Build history of the part. All positions in model axes, mm. Face numbers are marked on the shaded views. Round coordinates to 2 decimals unless told otherwise and drop trailing zeros. Order: outer loops, then holes, each group sorted by start corner. A loop starts at its lowest first (then second) coordinate and runs counter-clockwise, first axis right, second up. Notation, with made-up numbers: (1.25, 4.5) -> (46.25, 4.5) arc R16 ccw to (46.25, 12.5) -> close; hole circle Ø4 at (89.5, 53.25). An arc over 180 degrees is marked (long way). Use a Markdown table: item, result. Add a question column.
Item 1: Probe L1, parallel to Z at x = -71.5, y = 17; L2, parallel to Y at x = -71, z = 40.5; L3, parallel to X at y = 31, z = -36. List the from-to ranges inside material, lowest first.
Item 2: Two-plate mould, pull along Y, no slides. Class the marked faces 1, 2 and 3: released by +Y, released by -Y, zero draft, split by the parting line, or undercut.
Item 3: Slice it at B-B, the plane z = -17. Give the cut face in (x, y).
Item 4: Slice it at D-D, the plane z = -52. Give the cut face in (x, y), plus the area to 3 significant figures.
Item 5: Pin check, flat tips, straight feed: pin 1 (2 mm diameter, centred on x = -27.5, z = -48, fed in from -Y); pin 2 (4 mm diameter, centred on y = 40, z = -45.5, fed in from +X); pin 3 (4 mm diameter, centred on y = 40.5, z = -26.5, fed in from -X); pin 4 (23 mm diameter, centred on y = 45, z = -16, fed in from +X). Stop position of each tip, or through.
Item 6: Slice it at C-C, the plane y = 41. Give the cut face in (x, z).
Item 7: Slice it at A-A, the plane y = 4.5. Give the cut face in (x, z).
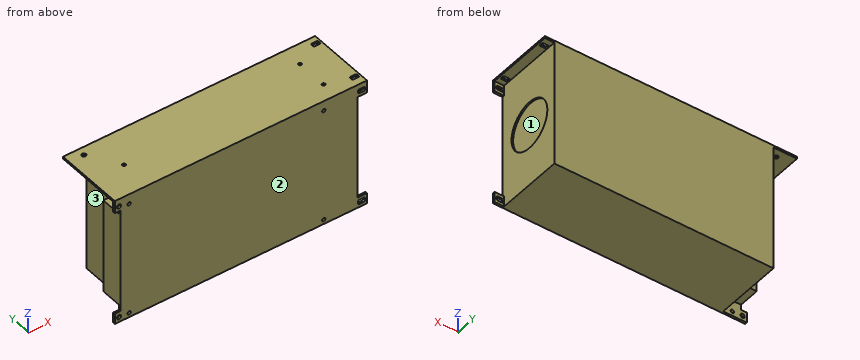
from build123d import *

# Parameters (mm, degrees)
SZKIC1_W                    = 240
SZKIC1_H                    = 122
DODANIE_WYCI_GNI_CIE1_DEPTH = 2
SZKIC2_W                    = 240
SZKIC2_H                    = 2
DODANIE_WYCI_GNI_CIE2_DEPTH = 64
SZKIC3_W                    = 9.1
SZKIC3_H                    = 99.9
SZKIC3_W_2                  = 5.5
WYTNIJ_WYCI_GNI_CIE1_DEPTH  = 180.195703173
SZKIC4_W                    = 208.5
SZKIC4_H                    = 120
DODANIE_WYCI_GNI_CIE3_DEPTH = 64
SZKIC5_R                    = 22.806294832
WYTNIJ_WYCI_GNI_CIE2_DEPTH  = 1.5
SZKIC6_W                    = 16.9
SZKIC6_H                    = 90.349503158
DODANIE_WYCI_GNI_CIE4_DEPTH = 20
WYTNIJ_WYCI_GNI_CIE3_DEPTH  = 180.195703173
SZKIC8_R                    = 2
WYTNIJ_WYCI_GNI_CIE4_DEPTH  = 180.195703173
SZKIC9_R                    = 1.6
SZKIC9_R_2                  = 1.651116854
WYTNIJ_WYCI_GNI_CIE5_DEPTH  = 2
SZKIC10_R                   = 2
WYTNIJ_WYCI_GNI_CIE6_DEPTH  = 2
SZKIC11_R                   = 1.455539738
SZKIC11_R_2                 = 1.5
WYTNIJ_WYCI_GNI_CIE7_DEPTH  = 2


with BuildPart() as part:
    # Szkic1 → Dodanie-wyciągnięcie1 (new body)
    with BuildSketch(Plane(origin=(0, 0, 0), x_dir=(1, 0, 0), z_dir=(0, 1, 0))):
        with Locations((29.433962264, 14.396226415)):
            Rectangle(SZKIC1_W, SZKIC1_H)
    extrude(amount=DODANIE_WYCI_GNI_CIE1_DEPTH)

    # Szkic2 → Dodanie-wyciągnięcie2 (add)
    with BuildSketch(Plane(origin=(0, 2, 0), x_dir=(1, 0, 0), z_dir=(0, 1, 0))):
        with Locations((29.433962264, -45.603773585)):
            Rectangle(SZKIC2_W, SZKIC2_H)
    extrude(amount=DODANIE_WYCI_GNI_CIE2_DEPTH)

    # Szkic3 → Wytnij-wyciągnięcie1 (cut, through all)
    with BuildSketch(Plane(origin=(0, 2, 0), x_dir=(1, 0, 0), z_dir=(0, 1, 0))):
        with Locations((144.883962264, 15.346226415)):
            Rectangle(SZKIC3_W, SZKIC3_H)
        with Locations((-87.816037736, 15.346226415)):
            Rectangle(SZKIC3_W_2, SZKIC3_H)
    extrude(amount=-WYTNIJ_WYCI_GNI_CIE1_DEPTH, mode=Mode.SUBTRACT)

    # Szkic4 → Dodanie-wyciągnięcie3 (add)
    with BuildSketch(Plane(origin=(0, 2, 0), x_dir=(1, 0, 0), z_dir=(0, 1, 0))):
        with Locations((36.083962264, 15.396226415)):
            Rectangle(SZKIC4_W, SZKIC4_H)
    extrude(amount=DODANIE_WYCI_GNI_CIE3_DEPTH)

    # Szkic5 → Wytnij-wyciągnięcie2 (cut)
    with BuildSketch(Plane(origin=(140.333962264, 0, 0), x_dir=(0, 0, -1), z_dir=(1, 0, 0))):
        with Locations((16.047891544, 34.239354483)):
            Circle(SZKIC5_R)
    extrude(amount=-WYTNIJ_WYCI_GNI_CIE2_DEPTH, mode=Mode.SUBTRACT)

    # Szkic6 → Dodanie-wyciągnięcie4 (add)
    with BuildSketch(Plane(origin=(0, 2, 0), x_dir=(1, 0, 0), z_dir=(0, 1, 0))):
        with Locations((-76.616037736, 15.234150699)):
            Rectangle(SZKIC6_W, SZKIC6_H)
    extrude(amount=DODANIE_WYCI_GNI_CIE4_DEPTH)

    # Szkic7 → Wytnij-wyciągnięcie3 (cut, through all)
    with BuildSketch(Plane(origin=(0, 2, 0), x_dir=(1, 0, 0), z_dir=(0, 1, 0))):
        with BuildLine():
            Line((141.913386631, 72.496226415), (146.454537897, 72.496226415))
            ThreePointArc((146.454537897, 72.496226415), (147.147095509, 72.20935966), (147.433962264, 71.516802048))
            Line((147.433962264, 71.516802048), (147.433962264, 69.275650782))
            ThreePointArc((147.433962264, 69.275650782), (147.147095509, 68.583093171), (146.454537897, 68.296226415))
            Line((146.454537897, 68.296226415), (141.913386631, 68.296226415))
            ThreePointArc((141.913386631, 68.296226415), (141.22082902, 68.583093171), (140.933962264, 69.275650782))
            Line((140.933962264, 69.275650782), (140.933962264, 71.516802048))
            ThreePointArc((140.933962264, 71.516802048), (141.22082902, 72.20935966), (141.913386631, 72.496226415))
        make_face()
        with BuildLine():
            Line((141.913386631, -37.603773585), (146.454537897, -37.603773585))
            ThreePointArc((146.454537897, -37.603773585), (147.147095509, -37.89064034), (147.433962264, -38.583197952))
            Line((147.433962264, -38.583197952), (147.433962264, -40.424349218))
            ThreePointArc((147.433962264, -40.424349218), (147.147095509, -41.116906829), (146.454537897, -41.403773585))
            Line((146.454537897, -41.403773585), (141.913386631, -41.403773585))
            ThreePointArc((141.913386631, -41.403773585), (141.22082902, -41.116906829), (140.933962264, -40.424349218))
            Line((140.933962264, -40.424349218), (140.933962264, -38.583197952))
            ThreePointArc((140.933962264, -38.583197952), (141.22082902, -37.89064034), (141.913386631, -37.603773585))
        make_face()
    extrude(amount=-WYTNIJ_WYCI_GNI_CIE3_DEPTH, mode=Mode.SUBTRACT)

    # Szkic8 → Wytnij-wyciągnięcie4 (cut, through all)
    with BuildSketch(Plane(origin=(0, 2, 0), x_dir=(1, 0, 0), z_dir=(0, 1, 0))):
        with Locations(Location((-86.566037736, 70.596226415, 0), (0, 0, 270))):
            Circle(SZKIC8_R)
        with Locations(Location((-86.566037736, -39.353773585, 0), (0, 0, 270))):
            Circle(SZKIC8_R)
    extrude(amount=-WYTNIJ_WYCI_GNI_CIE4_DEPTH, mode=Mode.SUBTRACT)

    # Szkic9 → Wytnij-wyciągnięcie5 (cut)
    with BuildSketch(Plane.XZ):
        with Locations(Location((-76.966037736, 37.203773585, 0), (0, 0, 270))):
            Circle(SZKIC9_R)
        with Locations(Location((108.333962264, 37.203773585, 0), (0, 0, 270))):
            Circle(SZKIC9_R)
        with Locations(Location((108.333962264, -70.996226415, 0), (0, 0, 270))):
            Circle(SZKIC9_R)
        with Locations(Location((-76.914920882, -71.047343269, 0), (0, 0, 270))):
            Circle(SZKIC9_R_2)
    extrude(amount=-WYTNIJ_WYCI_GNI_CIE5_DEPTH, mode=Mode.SUBTRACT)

    # Szkic10 → Wytnij-wyciągnięcie6 (cut)
    with BuildSketch(Plane.XY.offset(46.603773585)):
        with Locations((-76.566037736, 58.1)):
            Circle(SZKIC10_R)
        with BuildLine():
            Line((141.933962264, 60.3), (146.533962264, 60.3))
            ThreePointArc((146.533962264, 60.3), (147.241069045, 60.007106781), (147.533962264, 59.3))
            Line((147.533962264, 59.3), (147.533962264, 57.3))
            ThreePointArc((147.533962264, 57.3), (147.241069045, 56.592893219), (146.533962264, 56.3))
            Line((146.533962264, 56.3), (141.933962264, 56.3))
            ThreePointArc((141.933962264, 56.3), (141.226855483, 56.592893219), (140.933962264, 57.3))
            Line((140.933962264, 57.3), (140.933962264, 59.3))
            ThreePointArc((140.933962264, 59.3), (141.226855483, 60.007106781), (141.933962264, 60.3))
        make_face()
        with BuildLine():
            Line((141.933962264, 11.1), (146.533962264, 11.1))
            ThreePointArc((146.533962264, 11.1), (147.241069045, 10.807106781), (147.533962264, 10.1))
            Line((147.533962264, 10.1), (147.533962264, 8.1))
            ThreePointArc((147.533962264, 8.1), (147.241069045, 7.392893219), (146.533962264, 7.1))
            Line((146.533962264, 7.1), (141.933962264, 7.1))
            ThreePointArc((141.933962264, 7.1), (141.226855483, 7.392893219), (140.933962264, 8.1))
            Line((140.933962264, 8.1), (140.933962264, 10.1))
            ThreePointArc((140.933962264, 10.1), (141.226855483, 10.807106781), (141.933962264, 11.1))
        make_face()
    extrude(amount=-WYTNIJ_WYCI_GNI_CIE6_DEPTH, mode=Mode.SUBTRACT)

    # Szkic11 → Wytnij-wyciągnięcie7 (cut)
    with BuildSketch(Plane.XY.offset(46.603773585)):
        with Locations((120.133962264, 46.144460262)):
            Circle(SZKIC11_R)
        with Locations((120.088143939, 15.95)):
            Circle(SZKIC11_R_2)
        with Locations((-59.066037736, 30.5)):
            Circle(SZKIC11_R_2)
    extrude(amount=-WYTNIJ_WYCI_GNI_CIE7_DEPTH, mode=Mode.SUBTRACT)


solid = part.part
Check sheet entries:
| question | item | result |
|---|---|---|
| 1 | L1 | -60.41 to 29.94, 44.6 to 46.6 |
| 1 | L2 | 0 to 2 |
| 1 | L3 | -68.17 to 138.83 |
| 2 | face 1 | undercut |
| 2 | face 2 | released by -Y |
| 2 | face 3 | zero draft |
| 3 | outline | (-85.07, 0) -> (140.33, 0) -> (140.33, 11.45) -> (138.83, 11.45) -> (138.83, 57.03) -> (140.33, 57.03) -> (140.33, 66) -> (-68.17, 66) -> (-68.17, 22) -> (-85.07, 22) -> close |
| 4 | outline | (-85.07, 0) -> (140.33, 0) -> (140.33, 66) -> (-68.17, 66) -> (-68.17, 22) -> (-85.07, 22) -> close |
| 4 | area | 14,100 mm2 |
| 5 | pin 1 | y = 0 |
| 5 | pin 2 | x = 140.33 |
| 5 | pin 3 | x = -68.17 |
| 5 | pin 4 | x = 138.83 |
| 6 | outline | (-90.57, 44.6) -> (-68.17, 44.6) -> (-68.17, -75.4) -> (140.33, -75.4) -> (140.33, -37.83) -> (138.83, -37.83) -> (138.83, 5.73) -> (140.33, 5.73) -> (140.33, 44.6) -> (149.43, 44.6) -> (149.43, 46.6) -> (-90.57, 46.6) -> close |
| 7 | outline | (-90.57, 44.6) -> (-68.17, 44.6) -> (-68.17, 29.94) -> (-85.07, 29.94) -> (-85.07, -60.41) -> (-68.17, -60.41) -> (-68.17, -75.4) -> (140.33, -75.4) -> (140.33, 44.6) -> (149.43, 44.6) -> (149.43, 46.6) -> (-90.57, 46.6) -> close |
